```python
from build123d import *

# Parameters (mm, degrees)
F0_R      = 50
F1_DEPTH  = 71
F2_R      = 45
F3_DEPTH  = 65
F4_W      = 10.2
F4_H      = 6
F5_DEPTH  = 50
F6_W      = 10.2
F6_H      = 6
F7_DEPTH  = 50
F8_W      = 10.2
F8_H      = 6
F9_DEPTH  = 50
F10_W     = 10.2
F10_H     = 6
F11_DEPTH = 50
F12_R     = 5.6
F13_DEPTH = 55
F14_R     = 5.6
F15_DEPTH = 56
F17_DEPTH = 52
F18_DEPTH = 55
F19_R     = 45
F20_DEPTH = 50


with BuildPart() as f1:
    # F0 (on Top) → F1 (new body)
    with BuildSketch(Plane.XY):
        Circle(F0_R)
    extrude(amount=F1_DEPTH)

    # F2 (on face) → F3 (cut)
    with BuildSketch(Plane.XY.offset(71)):
        Circle(F2_R)
    extrude(amount=-F3_DEPTH, mode=Mode.SUBTRACT)

    # F4 (on Front) → F5 (cut)
    with BuildSketch(Plane.XZ):
        with Locations((0, 68)):
            Rectangle(F4_W, F4_H)
    extrude(amount=-F5_DEPTH, mode=Mode.SUBTRACT)

    # F6 (on Front) → F7 (cut)
    with BuildSketch(Plane.XZ):
        with Locations((0, 68)):
            Rectangle(F6_W, F6_H)
    extrude(amount=F7_DEPTH, mode=Mode.SUBTRACT)

    # F8 (on Right) → F9 (cut)
    with BuildSketch(Plane.YZ):
        with Locations((0, 68)):
            Rectangle(F8_W, F8_H)
    extrude(amount=-F9_DEPTH, mode=Mode.SUBTRACT)

    # F10 (on Right) → F11 (cut)
    with BuildSketch(Plane.YZ):
        with Locations((0, 68)):
            Rectangle(F10_W, F10_H)
    extrude(amount=F11_DEPTH, mode=Mode.SUBTRACT)

    # F12 (on Right) → F13 (cut)
    with BuildSketch(Plane.YZ):
        with Locations((0, 55.4)):
            Circle(F12_R)
    extrude(amount=-F13_DEPTH, mode=Mode.SUBTRACT)

    # F14 (on Right) → F15 (cut)
    with BuildSketch(Plane.YZ):
        with Locations((-6.6, 40.4)):
            Circle(F14_R)
        with Locations((6.6, 40.4)):
            Circle(F14_R)
    extrude(amount=F15_DEPTH, mode=Mode.SUBTRACT)

    # F16 (on Right) → F17 (join)
    with BuildSketch(Plane.YZ):
        with BuildLine():
            ThreePointArc((2.6579e-05, 36.4390160432), (0.7456952511, 38.2441613187), (1, 40.1806272566))
            ThreePointArc((1, 40.1806272566), (0.7456814951, 42.1171446646), (-2.6579e-05, 43.922330816))
            ThreePointArc((-2.6579e-05, 43.922330816), (-0.9999999998, 40.1806663261), (2.6579e-05, 36.4390160432))
        make_face()
        with BuildLine():
            ThreePointArc((-2.6579e-05, 43.922330816), (0.7456814951, 42.1171446646), (1, 40.1806272566))
            ThreePointArc((1, 40.1806272566), (0.7456952511, 38.2441613187), (2.6579e-05, 36.4390160432))
            ThreePointArc((2.6579e-05, 36.4390160432), (8.4365174079, 32.9350381074), (14, 40.1807196026))
            ThreePointArc((14, 40.1807196026), (8.4364659379, 47.4264148536), (-2.6579e-05, 43.922330816))
        make_face()
        with BuildLine():
            ThreePointArc((2.6579e-05, 36.4390160432), (-0.9999999998, 40.1806663261), (-2.6579e-05, 43.922330816))
            ThreePointArc((-2.6579e-05, 43.922330816), (-13.9999999998, 40.1805739801), (2.6579e-05, 36.4390160432))
        make_face()
    extrude(amount=F17_DEPTH)

    # F14 (on Right) → F18 (cut)
    with BuildSketch(Plane.YZ):
        with Locations((-6.6, 40.4)):
            Circle(F14_R)
        with Locations((6.6, 40.4)):
            Circle(F14_R)
    extrude(amount=F18_DEPTH, mode=Mode.SUBTRACT)

    # F19 (on face) → F20 (cut)
    with BuildSketch(Plane.XY.offset(6)):
        Circle(F19_R)
    extrude(amount=F20_DEPTH, mode=Mode.SUBTRACT)


solid = f1.part
```
The model under review builds one solid part; all positions refer to its coordinate system, in mm. A direction names the side the tool comes from. Round coordinates to 2 decimals unless told otherwise and drop trailing zeros. Loops run counter-clockwise (first coordinate to the right, second up) from the corner with the lowest first, then second, coordinate; pieces in that order, holes last. Notation, with made-up numbers: (-26, -14.75) - (17, -14.75) arc R31 ccw to (17, 14.25) - close; hole circle Ø5 at (-33, 82.5). An arc over 180 degrees is marked (long way). Use a Markdown table: item, result. Add a question column.
Q1. Add section D-D (y = -29). State the section outline as (x, z) points.
Q2. The part is to be moulded in two halves that separate along Y. For faces 1 (the face through (50.416, -13.995, 40.456)), 2 (the face through (-5.1, 47, 68)), 3 (the face through (-47, -5.1, 68)), say which applies: pulls with the +Y half, pulls with the -Y half, needs draft (parallel to the pull), parting line crosses it, or undercut.
Q3. Add section A-A (y = 9). State the section outline as (x, z) points.
Q4. For probe 1 along Y at (x, z) = (0, 61.75); probe 2 along Z at (x, y) = (-47.05, 0); probe 3 along Z at (x, y) = (37, -6), list the stretches that pass through material, from the lowest coordinate up.
Q5. Insertion check: pin 1 Ø5 at (x, z) = (10, 62) entering from +Y; pin 2 Ø4 at (x, z) = (48, 67) entering from +Y; pin 3 Ø8 at (x, z) = (31.5, 26.5) entering from -Y. Each pin has a flat end and moves straight along its axis. Give the tip position at first contact, or say it passes through.
Q6. Add section B-B (z = 40.4). State the section outline as (x, y) points, plus the area to 3 significant figures.
Q7. Machinability: for faces 4 (the face through (48.56, 11.94, 42.08)), 5 (the face through (-1, 1, 6)), 6 (the face through (32, 32, 71)), 7 (the face through (5.1, 47, 68)), 8 (the face through (-47, 0, 65)), which of the approach directions +Z, -Z, +X, -X, +Y, -Y give a long, thin tool a straight path to every point of the face, cutting with its end or side? Answer none if there is none.
Q8. Add section C-C (x = 0). State the section outline as (y, z) points.
Worked answers:
| question | item | result |
|---|---|---|
| 1 | outline | (-40.73, 0) - (40.73, 0) - (40.73, 71) - (34.41, 71) - (34.41, 6) - (-34.41, 6) - (-34.41, 71) - (-40.73, 71) - close |
| 2 | face 1 | undercut |
| 2 | face 2 | needs draft |
| 2 | face 3 | undercut |
| 3 | outline | (-49.18, 0) - (49.18, 0) - (49.18, 33.11) - (52, 33.11) - (52, 35.34) - (44.09, 35.34) - (44.09, 6) - (-44.09, 6) - (-44.09, 71) - (-49.18, 71) - close; (44.09, 45.46) - (52, 45.46) - (52, 47.25) - (49.18, 47.25) - (49.18, 71) - (44.09, 71) - close |
| 4 | probe 1 | -50 to -45, 45 to 50 |
| 4 | probe 2 | 0 to 49.8, 61 to 65 |
| 4 | probe 3 | 0 to 6 |
| 5 | pin 1 | y = 49.43 |
| 5 | pin 2 | y = 19.6 |
| 5 | pin 3 | y = -41.76 |
| 6 | outline | (43.31, -12.2) arc R45 cw (long way) to (43.31, 12.2) - (52, 12.2) - (52, 14) - (48, 14) arc R50 ccw (long way) to (48, -14) - (52, -14) - (52, -12.2) - close; (44.99, -1) - (52, -1) - (52, 1) - (44.99, 1) arc R45 cw to start |
| 6 | area | 1,400 mm² |
| 7 | face 4 | +X |
| 7 | face 5 | +Z |
| 7 | face 6 | +Z, +X, -X, +Y, -Y |
| 7 | face 7 | +Z, +Y, -Y |
| 7 | face 8 | +Z, +X, -X |
| 8 | outline | (-50, 0) - (50, 0) - (50, 65) - (45, 65) - (45, 6) - (-45, 6) - (-45, 65) - (-50, 65) - close |
